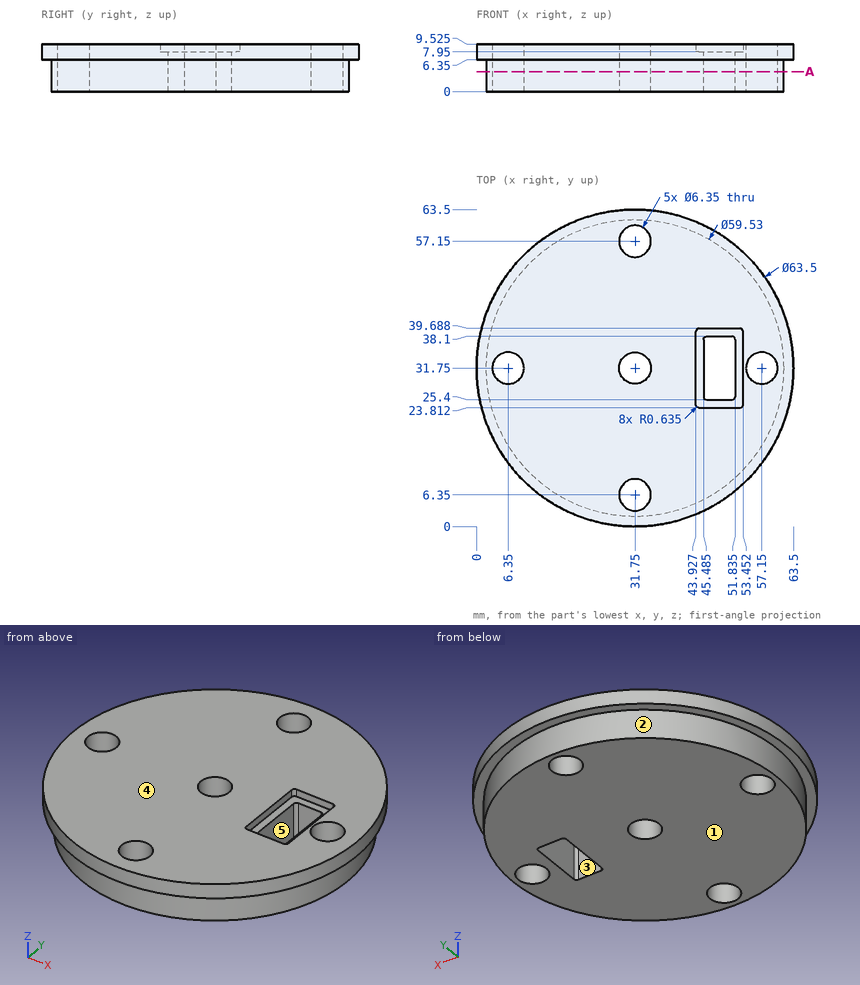
Study the drawing (mm; zero at the part's minimum x, y, z) and answer. A direction names the side the tool comes from. Round coordinates to 2 decimals unless told otherwise and drop trailing zeros. Return JSON: item names as keys, results as strings. Group by question number.
Q1. The mould has two halves that part along Y. Classify the marked faces 1, 2 and 3: released by +Y, released by -Y, zero draft, split by the parting line, or undercut.
Q2. Find the intervals of material crossed by L1, parallel to Y at x = 31.75, z = 4.75 (1 decimal); L2, parallel to X at y = 31.5, z = 1.5 (1 decimal); L3, parallel to Y at x = 57.15, z = 5.25 (1 decimal), in increasing order.
Q3. For the marked faces 4 and 5, determine the directions among +Z, -Z, +X, -X, +Y, -Y from which every point of the face is accessible in a straight line to the end or side of a thin tool.
Q4. The part is cut by section A-A on z = 4. Count the separate pieces of the cut face and the enclosed holes in it.
Q5. Each of these flat-tipped pins is pushed along its axis until it touches: pin 1 Ø3 at (y, z) = (18.5, 8) entering from +X (1 decimal); pin 2 Ø0.5 at (y, z) = (30, 8.5) entering from +X (1 decimal); pin 3 Ø1.5 at (x, z) = (49.5, 3.5) entering from +Y; pin 4 Ø4 at (x, y) = (31.75, 57.15) entering from +Z. Where does it stop, or does it pass through?
Solved:
{
 "1": {"face 1": "zero draft", "face 2": "split by the parting line", "face 3": "undercut"},
 "2": {"L1": "2 to 3.2, 9.5 to 28.6, 34.9 to 54, 60.3 to 61.5", "L2": "2 to 3.2, 9.5 to 28.6, 34.9 to 45.5, 51.8 to 54, 60.3 to 61.5", "L3": "16.2 to 28.6, 34.9 to 47.3"},
 "3": {"face 4": "+Z, +X, -X, +Y, -Y", "face 5": "+Z, -Z"},
 "4": {"separate pieces": "1", "enclosed holes": "6"},
 "5": {"pin 1": "x = 61.2", "pin 2": "x = 63.5", "pin 3": "y = 56.18", "pin 4": "through"}
}
